CAD build for the part. Positions are in the model's coordinates, mm. A direction names the side the tool comes from. Coordinates: 2 decimals unless noted, no trailing zeros. Loops run counter-clockwise (first coordinate to the right, second up) from the corner with the lowest first, then second, coordinate; pieces in that order, holes last. Notation, with made-up numbers: (48.5, 78) -> (63.5, 78) arc R23 ccw to (63.5, 109) -> close; hole circle Ø2 at (-21, 73). An arc over 180 degrees is marked (long way). Write item = value, one per line. Start each with the question number.
(1) Band-saw the part on A-A (y = 0). Write the cut outline in (x, z) (1 decimal), and give its area (3 significant figures).
(2) Drill centre lines: line 1 (X direction, y = 0, z = 62) (1 decimal); line 2 (X direction, y = 0, z = 11); line 3 (Z direction, x = -26.5, y = -11.5) (3 decimals). Where is each one in solid material? Low to high. Write a range as from..to.
(3) Flat gauge pins, fed straight in: P1, Ø1, axis at y = -2.5, z = 60.5, coming from the -X side; P2, Ø1, axis at y = -28.5, z = 23, coming from the -X side (3 decimals); P3, Ø12, axis at x = -22, z = 52.5, coming from the +Y side; P4, Ø12, axis at x = -12, y = 34.5, coming from the -Z side. Where does each tip first touch, or does it go through?
(4) Pull direction X, two halves, no side cores. Call faces 4 (the face through (-2.3, 35.26, 36.06)), 5 (the face through (-54.882, -34.991, 51.156)), 6 (the face through (58, -19, 76.2)): +X half, -X half, draft (parallel to the pull), parting line (faces both ways), or undercut.
(5) Band-saw the part on D-D (x = -50.5). Write the cut outline in (y, z) (3 decimals), and give its area (3 significant figures).
(6) Tool access for faces 1 (the face through (-36.48, 39.78, 39.71)), 2 (the face through (-3.62, 21.88, 16.65)), 3 (the face through (28, -1, 25.4)): list every direction of +Z, -Z, +X, -X, +Y, -Y with a clear straight run to the whole face (end or side of a thin tool).
(7) Band-saw the part on B-B (x = 0). Count the separate pieces of the cut face and the enclosed holes in it, and give its area (3 significant figures).
```python
from build123d import *

# Parameters (mm, degrees)
ESQUISSE3_R                                       = 18.25625
ENL_V_MAT_EXTRU_1_DEPTH                           = 120.495628843
FRAISAGE_POUR_VIS_T_TE_FRAIS_E_BOMB_E_D           = 9.525
FRAISAGE_POUR_VIS_T_TE_FRAIS_E_BOMB_E_CSINK_D     = 19.05
FRAISAGE_POUR_VIS_T_TE_FRAIS_E_BOMB_E_CSINK_ANGLE = 82
R_P_TITION_CIRCULAIRE1_COUNT                      = 3
CHANFREIN1_SIZE                                   = 1.5875
ESQUISSE7_W                                       = 5.35813
ESQUISSE7_H                                       = 65.0875


with BuildPart() as part:
    # Esquisse2 → Révolution2 (revolve)
    with BuildSketch(Plane(origin=(0, 0, 0), x_dir=(0, 0, -1), z_dir=(1, 0, 0)), mode=Mode.PRIVATE) as r_volution2_sk:
        Polygon((0, 0), (0, 26.19375), (-25.4, 26.19375), (-25.4, 65.0875), (-76.2, 65.0875), (-76.2, 60.325), (-38.1, 60.325), (-38.1, 53.975), (-41.275, 53.975), (-41.275, 0), align=None)
    revolve(r_volution2_sk.sketch.rotate(Axis((0, 0, 41.275), (0, 0, -1)), 180), axis=Axis((0, 0, 41.275), (0, 0, -1)))

    # Esquisse3 → Enlèv. mat.-Extru.1 (cut, through all)
    with BuildSketch(Plane(origin=(0, 0, 0), x_dir=(-1, 0, 0), z_dir=(0, 0, -1))):
        with Locations(Location((0, 0, 0), (0, 0, 90))):
            Circle(ESQUISSE3_R)
    extrude(amount=-ENL_V_MAT_EXTRU_1_DEPTH, mode=Mode.SUBTRACT)

    # Fraisage pour vis à tête fraisée bombée 3/81 (through all)
    with Locations(Plane.XY.offset(41.275)):
        with Locations((0, 39.6875)):
            fraisage_pour_vis_t_te_frais_e_bomb_e = CounterSinkHole(FRAISAGE_POUR_VIS_T_TE_FRAIS_E_BOMB_E_D / 2, FRAISAGE_POUR_VIS_T_TE_FRAIS_E_BOMB_E_CSINK_D / 2, counter_sink_angle=FRAISAGE_POUR_VIS_T_TE_FRAIS_E_BOMB_E_CSINK_ANGLE)

    # Répétition circulaire1: Fraisage pour vis à tête fraisée bombée 3/81 ×3 about axis
    r_p_tition_circulaire1_axis = Axis((0, 0, 0), (0, 0, 1))
    for i in range(1, R_P_TITION_CIRCULAIRE1_COUNT):
        add(fraisage_pour_vis_t_te_frais_e_bomb_e.rotate(r_p_tition_circulaire1_axis, i * 360 / R_P_TITION_CIRCULAIRE1_COUNT), mode=Mode.SUBTRACT)

    # Chanfrein1
    chanfrein1_edges = [part.edges().sort_by_distance(p)[0] for p in [
        (0, 26.19375, 0),
    ]]
    chamfer(chanfrein1_edges, length=CHANFREIN1_SIZE)

    # Esquisse7 → Trou taraudé 1/2-131 (revolve, cut)
    with BuildSketch(Plane(origin=(0, 0, 12.7), x_dir=(0, 0, -1), z_dir=(1, 0, 0))):
        with Locations((2.679065, 32.54375)):
            Rectangle(ESQUISSE7_W, ESQUISSE7_H)
    revolve(axis=Axis((0, -6.35, 12.7), (0, 1, 0)), mode=Mode.SUBTRACT)


solid = part.part
```
Findings below:
q1.outline = (-65.1, 25.4) -> (-26.2, 25.4) -> (-26.2, 1.6) -> (-24.6, 0) -> (-18.3, 0) -> (-18.3, 41.3) -> (-54, 41.3) -> (-54, 38.1) -> (-60.3, 38.1) -> (-60.3, 76.2) -> (-65.1, 76.2) -> close; (18.3, 0) -> (24.6, 0) -> (26.2, 1.6) -> (26.2, 25.4) -> (65.1, 25.4) -> (65.1, 76.2) -> (60.3, 76.2) -> (60.3, 38.1) -> (54, 38.1) -> (54, 41.3) -> (18.3, 41.3) -> close
q1.area = 2,180 mm²
q2.line_1 = -65.1..-60.3, 60.3..65.1
q2.line_2 = -26.19..-18.26, 18.26..26.19
q2.line_3 = 25.4..41.275
q3.P1 = -65.06
q3.P2 = through
q3.P3 = 63.09
q3.P4 = 25.4
q4.face_4 = undercut
q4.face_5 = parting line
q4.face_6 = draft
q5.outline = (-41.063, 25.4) -> (41.063, 25.4) -> (41.063, 76.2) -> (32.998, 76.2) -> (32.998, 38.1) -> (19.054, 38.1) -> (19.054, 41.275) -> (-19.054, 41.275) -> (-19.054, 38.1) -> (-32.998, 38.1) -> (-32.998, 76.2) -> (-41.063, 76.2) -> close
q5.area = 1,780 mm²
q6.face_1 = +Z
q6.face_2 = +Y
q6.face_3 = -Z
q7.separate_pieces = 4
q7.enclosed_holes = 0
q7.area = 1,920 mm²
